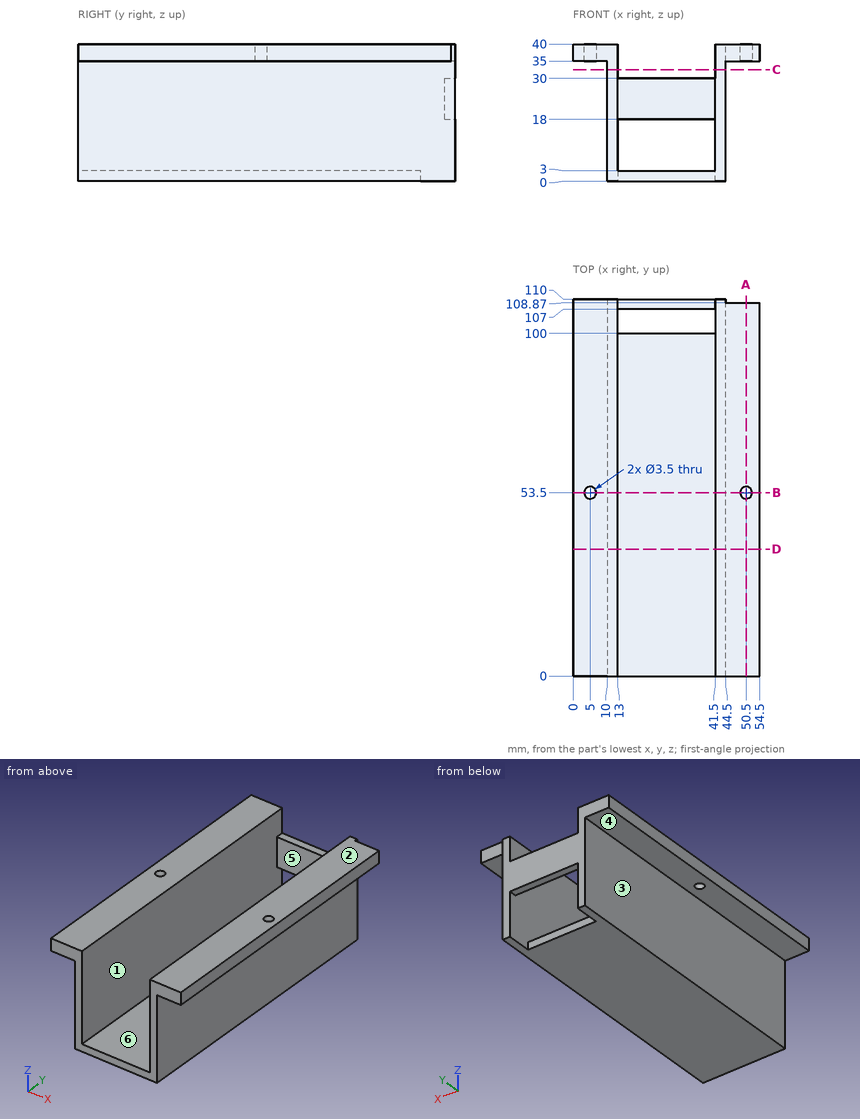
For this review, use the dimensioned drawing (mm, ordinates from the lowest corner) and the shaded views. A direction names the side the tool comes from. Give positions to 0.01 mm unless a question says otherwise; leave off trailing zeros. Write each loop counter-clockwise with the first axis right and the second up, starting at its lowest first coordinate (ties: lowest second). Pieces come first, ordered by that corner, then holes. Notation, with made-up numbers: M 13,-17 L 35,-17 A25 cw 35,-4 Z; hole C -14.5,9 d5. An arc over 180 degrees is marked long. Answer as a JSON object with one key per item and string values. Group by question number.
1) Clearance check with flat-ended pins moving along their axes: pin 1 Ø4 at (y, z) = (32.5, 11) entering from -X; pin 2 Ø2.5 at (x, y) = (20.5, 108) entering from -Z; pin 3 Ø8 at (x, z) = (24, 6.5) entering from -Y; pin 4 Ø5 at (x, z) = (16, 30.5) entering from -Y. State where each tip first meets the part, or that it passes through.
2) We need section C-C (z = 32.5). Give the boundary of the cut face in (x, y).
3) We need section A-A (x = 50.5). Give the boundary of the cut face in (y, z).
4) We need section B-B (y = 53.5). Give the boundary of the cut face in (x, z).
5) For line 1 along X through (y, z) = (88.5, 34.5); line 2 along Y through (x, z) = (5, 37); line 3 along Z through (x, y) = (27.5, 30), list the stretches that pass through material, from the lowest coordinate up.
6) We need section D-D (y = 37). Give the boundary of the cut face in (x, z).
7) Mouldability with a two-part tool opening along X and no side actions: class the marked faces 1, 2 and 3 as released by +X, released by -X, zero draft, split by the parting line, or undercut.
8) Tool access review of the marked faces 4, 5 and 6: name each direction out of +Z, -Z, +X, -X, +Y, -Y from which nothing blocks a thin tool from reaching the whole face with its end or side.
Answer key:
{
 "1": {"pin 1": "stops at x = 10", "pin 2": "stops at z = 18", "pin 3": "stops at y = 0", "pin 4": "stops at y = 107"},
 "2": {"outline": "M 10,0 L 13,0 L 13,110 L 10,110 Z; M 41.5,0 L 44.5,0 L 44.5,110 L 41.5,110 Z"},
 "3": {"outline": "M 0,35 L 51.75,35 L 51.75,40 L 0,40 Z; M 55.25,35 L 108.87,35 L 108.87,40 L 55.25,40 Z"},
 "4": {"outline": "M 0,35 L 3.25,35 L 3.25,40 L 0,40 Z; M 6.75,35 L 10,35 L 10,0 L 44.5,0 L 44.5,35 L 48.75,35 L 48.75,40 L 41.5,40 L 41.5,3 L 13,3 L 13,40 L 6.75,40 Z; M 52.25,35 L 54.5,35 L 54.5,40 L 52.25,40 Z"},
 "5": {"line 1": "x = 10 to 13, 41.5 to 44.5", "line 2": "y = 0 to 51.75, 55.25 to 110", "line 3": "z = 0 to 3"},
 "6": {"outline": "M 0,35 L 10,35 L 10,0 L 44.5,0 L 44.5,35 L 54.5,35 L 54.5,40 L 41.5,40 L 41.5,3 L 13,3 L 13,40 L 0,40 Z"},
 "7": {"face 1": "undercut", "face 2": "zero draft", "face 3": "released by -X"},
 "8": {"face 4": "-Z, -X, +Y, -Y", "face 5": "+Z, -Z, -Y", "face 6": "+Z, +Y, -Y"}
}
